from build123d import *

# Parameters (mm, degrees)
F0_R     = 60
F1_DEPTH = 85
F2_T     = -10
F3_R     = 14.5
F4_DEPTH = 25


with BuildPart() as f1:
    # F0 (on Top) → F1 (new body, symmetric)
    with BuildSketch(Plane.XY):
        Circle(F0_R)
    extrude(amount=F1_DEPTH, both=True)

    # F2
    f2_openings = [f1.faces().sort_by_distance(p)[0] for p in [
        (0, 0, 85),
    ]]
    offset(amount=F2_T, openings=f2_openings)

    # F3 (on face) → F4 (cut, symmetric)
    with BuildSketch(Plane(origin=(0, 0, -85), x_dir=(1, 0, 0), z_dir=(0, 0, -1))):
        Circle(F3_R)
    extrude(amount=F4_DEPTH, both=True, mode=Mode.SUBTRACT)


solid = f1.part
Work out the finished part from the listing and answer in its coordinate system (mm). A direction names the side the tool comes from. Give positions to 0.01 mm unless a question says otherwise; leave off trailing zeros. Write each loop counter-clockwise with the first axis right and the second up, starting at its lowest first coordinate (ties: lowest second). Pieces come first, ordered by that corner, then holes.
Q1. Given pin 1 (3 mm diameter, centred on y = 30.5, z = -60.5, fed in from -X); pin 2 (1 mm diameter, centred on x = 31, y = 2, fed in from +Z); pin 3 (8 mm diameter, centred on y = 37, z = 50, fed in from +X), each flat-ended and moving along its own axis, determine where each tip first touches the part or whether it passes through.
Answer:
pin 1: stops at x = -52.53
pin 2: stops at z = -75
pin 3: stops at x = 50.11
Q2. The part is cut by section D-D on y = -19. Give the vertices of the cut face in (x, z).
Answer:
outline: (-56.91, -85) - (56.91, -85) - (56.91, 85) - (46.25, 85) - (46.25, -75) - (-46.25, -75) - (-46.25, 85) - (-56.91, 85) - close
Q3. For a pull along Y with two mould halves and no side action, classify faces 1 (the face through (-59.94, 2.64, 1.19)), 2 (the face through (12, -12, -85)), 3 (the face through (47.69, 15.02, 6.12)) as released by +Y, released by -Y, zero draft, split by the parting line, or undercut.
Answer:
face 1: split by the parting line
face 2: zero draft
face 3: undercut
Q4. The part is cut by section C-C on x = -48. Give the vertices of the cut face in (y, z), and give its area (3 significant figures).
Answer:
outline: (-36, -85) - (36, -85) - (36, 85) - (14, 85) - (14, -75) - (-14, -75) - (-14, 85) - (-36, 85) - close
area: 7,760 mm2
Q5. Straight lines are drawn through the part: L1, parallel to Y at x = -2, z = 42; L2, parallel to Y at x = 0, z = -78; L3, parallel to Z at x = -12, y = -36.5. For each, find the intervals that lie inside material, in ascending order.
Answer:
L1: y = -59.97 to -49.96, 49.96 to 59.97
L2: y = -60 to -14.5, 14.5 to 60
L3: z = -85 to -75
Q6. A tool of negligible diameter and unlimited length cuts with its end or side. For faces 4 (the face through (10.4, -10.4, -75)), 5 (the face through (-23, 45, 85)), from which of +Z, -Z, +X, -X, +Y, -Y can it reach the whole face along a straight path? Write none if from no direction.
Answer:
face 4: +Z
face 5: +Z, +X, -X, +Y, -Y
Q7. The part is cut by section A-A on y = 0. Give the vertices of the cut face in (x, z).
Answer:
outline: (-60, -85) - (-14.5, -85) - (-14.5, -75) - (-50, -75) - (-50, 85) - (-60, 85) - close; (14.5, -85) - (60, -85) - (60, 85) - (50, 85) - (50, -75) - (14.5, -75) - close
